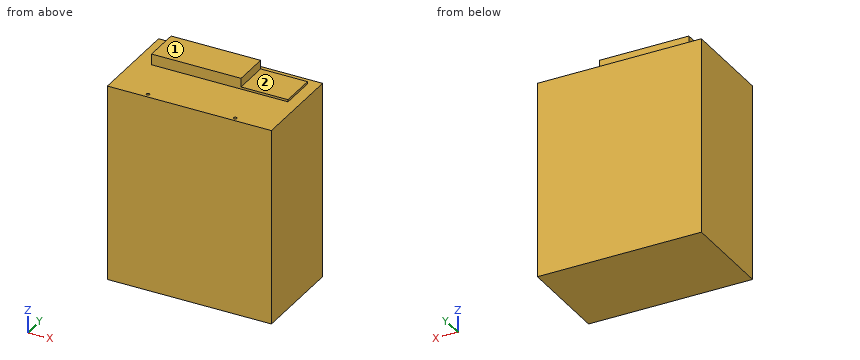
from build123d import *

# Parameters (mm, degrees)
SKETCH1_W           = 150.3
SKETCH1_H           = 86.5
BOSS_EXTRUDE1_DEPTH = 180
SKETCH1_3_R         = 1.47
CUT_EXTRUDE1_DEPTH  = 10
SKETCH1_4_W         = 82
SKETCH1_4_H         = 33
BOSS_EXTRUDE2_DEPTH = 10
SKETCH1_5_W         = 43
SKETCH1_5_H         = 33
BOSS_EXTRUDE3_DEPTH = 2


with BuildPart() as part:
    # Sketch1 → Boss-Extrude1 (new body)
    with BuildSketch(Plane.XY):
        with Locations((75.15, 43.25)):
            Rectangle(SKETCH1_W, SKETCH1_H)
    extrude(amount=-BOSS_EXTRUDE1_DEPTH)

    # Sketch1<3> → Cut-Extrude1 (cut)
    with BuildSketch(Plane.XY):
        with Locations((35.15, 3.89)):
            Circle(SKETCH1_3_R)
        with Locations((115.15, 3.89)):
            Circle(SKETCH1_3_R)
    extrude(amount=-CUT_EXTRUDE1_DEPTH, mode=Mode.SUBTRACT)

    # Sketch1<4> → Boss-Extrude2 (add)
    with BuildSketch(Plane.XY):
        with Locations((56, 63.5)):
            Rectangle(SKETCH1_4_W, SKETCH1_4_H)
    extrude(amount=BOSS_EXTRUDE2_DEPTH)

    # Sketch1<5> → Boss-Extrude3 (add)
    with BuildSketch(Plane.XY):
        with Locations((118.5, 63.5)):
            Rectangle(SKETCH1_5_W, SKETCH1_5_H)
    extrude(amount=BOSS_EXTRUDE3_DEPTH)


solid = part.part
Geometry check sheet. Reference: the model listing, model coordinates, mm. Face numbers are marked on the shaded views. A direction names the side the tool comes from. Give positions to 0.01 mm unless a question says otherwise; leave off trailing zeros. Loops run counter-clockwise (first coordinate to the right, second up) from the corner with the lowest first, then second, coordinate; pieces in that order, holes last. Notation, with made-up numbers: M 17.25,-32 L 30.25,-32 A18 ccw 30.25,-17 Z; hole C 89,24.25 d4. An arc over 180 degrees is marked long. Write each question's results on one line, items separated by ' | '.
1) Section check B-B, the plane x = 72.5. Record the boundary of the cut face in (y, z).
Answers follow:
outline: M 0,-180 L 86.5,-180 L 86.5,0 L 80,0 L 80,10 L 47,10 L 47,0 L 0,0 Z
2) Thickness scan on line 1 (Y direction, x = 115.15, z = -3.25); line 2 (X direction, y = 3, z = -6); line 3 (Z direction, x = 130.5, y = 63). Record the ranges inside material, lowest first.
Answers follow:
line 1: 0 to 2.42, 5.36 to 86.5 | line 2: 0 to 33.98, 36.32 to 113.98, 116.32 to 150.3 | line 3: -180 to 2
3) Gauge pin test, flat ends, axial feed: pin 1 (8 mm diameter, centred on x = 81.5, y = 38, fed in from +Z); pin 2 (16.5 mm diameter, centred on x = 122.5, y = 60.5, fed in from +Z); pin 3 (1.6 mm diameter, centred on y = 63, z = 1, fed in from +X). Record the tip position at first contact, or that the pin passes through.
Answers follow:
pin 1: z = 0 | pin 2: z = 2 | pin 3: x = 140
4) Tool access check on the marked faces 1 and 2. Record the directions out of +Z, -Z, +X, -X, +Y, -Y that give a thin tool (end or side, any length) a straight path to the whole face; none if there is none.
Answers follow:
face 1: +Z, +X, -X, +Y, -Y | face 2: +Z, +X, +Y, -Y
5) Section check C-C, the plane y = 14. Record the boundary of the cut face in (x, z).
Answers follow:
outline: M 0,-180 L 150.3,-180 L 150.3,0 L 0,0 Z
6) Section check A-A, the plane y = 70. Record the boundary of the cut face in (x, z).
Answers follow:
outline: M 0,-180 L 150.3,-180 L 150.3,0 L 140,0 L 140,2 L 97,2 L 97,10 L 15,10 L 15,0 L 0,0 Z
